Check sheet for the modelled part. Datum: model origin and axes. Units: mm. Round coordinates to 2 decimals unless told otherwise and drop trailing zeros. Answer in a Markdown table with one row per item.
```python
from build123d import *
from OCP.BRepFilletAPI import BRepFilletAPI_MakeChamfer

# Parameters (mm, degrees)
SKETCH1_W                       = 140
SKETCH1_H                       = 80
BOSS_EXTRUDE1_DEPTH             = 7
SKETCH3_W                       = 140
SKETCH3_H                       = 80
SKETCH2_W                       = 120
SKETCH2_H                       = 60
CHAMFER1_SIZE                   = 2
SKETCH4_R                       = 2.05
CUT_EXTRUDE1_DEPTH              = 7
SKETCH5_W                       = 114
SKETCH5_H                       = 50
CUT_EXTRUDE2_DEPTH              = 29
SKETCH6_W                       = 114
SKETCH6_H                       = 62
CUT_EXTRUDE3_DEPTH              = 25
SKETCH7_W                       = 6
SKETCH7_H                       = 62
CUT_EXTRUDE4_DEPTH              = 4
SKETCH8_R                       = 2.05
CUT_EXTRUDE5_DEPTH              = 6
CHAMFER2_SIZE                   = 1
CHAMFER2_SIZE2                  = 0.471497246
CHAMFER3_SIZE                   = 0.6
SKIZZE1_W                       = 54.050484576
SKIZZE1_H                       = 7.5
SKIZZE1_W_2                     = 4
SKIZZE1_H_2                     = 21.453027382
AUFSATZ_LINEAR_AUSTRAGEN1_DEPTH = 10
SKIZZE3_W                       = 29.974757712
SKIZZE3_H                       = 3
SCHNITT_LINEAR_AUSTRAGEN2_DEPTH = 4


with BuildPart() as part:
    # Sketch1 → Boss-Extrude1 (new body)
    with BuildSketch(Plane(origin=(0, 0, 0), x_dir=(1, 0, 0), z_dir=(0, 1, 0))):
        Rectangle(SKETCH1_W, SKETCH1_H)
    extrude(amount=BOSS_EXTRUDE1_DEPTH)

    # Sketch3 → Loft2 section 0
    with BuildSketch(Plane(origin=(0, 7, 0), x_dir=(1, 0, 0), z_dir=(0, 1, 0))):
        Rectangle(SKETCH3_W, SKETCH3_H)
    # Sketch2 → Loft2 section 1
    with BuildSketch(Plane(origin=(0, 30, 0), x_dir=(1, 0, 0), z_dir=(0, 1, 0))):
        Rectangle(SKETCH2_W, SKETCH2_H)
    loft()

    # Chamfer1
    chamfer1_edges = [part.edges().sort_by_distance(p)[0] for p in [
        (-70, 3.5, 40),
        (70, 3.5, 40),
        (70, 3.5, -40),
        (-70, 3.5, -40),
    ]]
    chamfer(chamfer1_edges, length=CHAMFER1_SIZE)

    # Sketch4 → Cut-Extrude1 (cut)
    with BuildSketch(Plane.XZ):
        with Locations(Location((40, -36.5, 0), (0, 0, 270))):
            Circle(SKETCH4_R)
        with Locations(Location((-40, -36.5, 0), (0, 0, 270))):
            Circle(SKETCH4_R)
    cut_extrude1 = extrude(amount=-CUT_EXTRUDE1_DEPTH, mode=Mode.SUBTRACT)

    # Sketch5 → Cut-Extrude2 (cut)
    with BuildSketch(Plane.XZ):
        Rectangle(SKETCH5_W, SKETCH5_H)
    extrude(amount=-CUT_EXTRUDE2_DEPTH, mode=Mode.SUBTRACT)

    # Mirror1: Cut-Extrude1 across plane
    add(cut_extrude1.mirror(Plane.XY), mode=Mode.SUBTRACT)

    # Sketch6 → Cut-Extrude3 (cut)
    with BuildSketch(Plane.XZ):
        Rectangle(SKETCH6_W, SKETCH6_H)
    extrude(amount=-CUT_EXTRUDE3_DEPTH, mode=Mode.SUBTRACT)

    # Sketch7 → Cut-Extrude4 (cut)
    with BuildSketch(Plane.XZ):
        with Locations((-60, 0)):
            Rectangle(SKETCH7_W, SKETCH7_H)
        with Locations((60, 0)):
            Rectangle(SKETCH7_W, SKETCH7_H)
    extrude(amount=-CUT_EXTRUDE4_DEPTH, mode=Mode.SUBTRACT)

    # Sketch8 → Cut-Extrude5 (cut)
    with BuildSketch(Plane.XZ.offset(-4)):
        with Locations(Location((-60, 25, 0), (0, 0, 270))):
            Circle(SKETCH8_R)
        with Locations(Location((-60, -25, 0), (0, 0, 270))):
            Circle(SKETCH8_R)
        with Locations(Location((60, -25, 0), (0, 0, 90))):
            Circle(SKETCH8_R)
        with Locations(Location((60, 25, 0), (0, 0, 90))):
            Circle(SKETCH8_R)
    extrude(amount=-CUT_EXTRUDE5_DEPTH, mode=Mode.SUBTRACT)

    # Chamfer2: one chamfer whose edges measure the first distance from different faces: ONE call of the kernel's chamfer builder (chamfer() names one face for all edges)
    chamfer2_edges_1 = [part.edges().sort_by_distance(p)[0] for p in [
        (60, 30, 0),
    ]]
    chamfer2_side_1 = [part.faces().sort_by_distance(p)[0] for p in [
        (65.225405922, 17.98156638, 0),
    ]]
    chamfer2_edges_2 = [part.edges().sort_by_distance(p)[0] for p in [
        (0, 30, -30),
    ]]
    chamfer2_side_2 = [part.faces().sort_by_distance(p)[0] for p in [
        (0, 18.221212121, -35.121212121),
    ]]
    chamfer2_edges_3 = [part.edges().sort_by_distance(p)[0] for p in [
        (-60, 30, 0),
    ]]
    chamfer2_side_3 = [part.faces().sort_by_distance(p)[0] for p in [
        (-65.225405922, 17.98156638, 0),
    ]]
    chamfer2_edges_4 = [part.edges().sort_by_distance(p)[0] for p in [
        (0, 30, 30),
    ]]
    chamfer2_side_4 = [part.faces().sort_by_distance(p)[0] for p in [
        (0, 18.221212121, 35.121212121),
    ]]
    chamfer2 = BRepFilletAPI_MakeChamfer(part.part.solid().wrapped)
    for e in chamfer2_edges_1:
        chamfer2.Add(CHAMFER2_SIZE, CHAMFER2_SIZE2, e.wrapped, chamfer2_side_1[0].wrapped)  # the first distance lies on this face
    for e in chamfer2_edges_2:
        chamfer2.Add(CHAMFER2_SIZE, CHAMFER2_SIZE2, e.wrapped, chamfer2_side_2[0].wrapped)  # the first distance lies on this face
    for e in chamfer2_edges_3:
        chamfer2.Add(CHAMFER2_SIZE, CHAMFER2_SIZE2, e.wrapped, chamfer2_side_3[0].wrapped)  # the first distance lies on this face
    for e in chamfer2_edges_4:
        chamfer2.Add(CHAMFER2_SIZE, CHAMFER2_SIZE2, e.wrapped, chamfer2_side_4[0].wrapped)  # the first distance lies on this face
    add(Compound.cast(chamfer2.Shape()), mode=Mode.REPLACE)

    # Chamfer3
    chamfer3_edges = [part.edges().sort_by_distance(p)[0] for p in [
        (0, 0, 40),
        (70, 0, 0),
        (-70, 0, 0),
        (0, 0, -40),
        (-69, 0, -39),
        (69, 0, -39),
        (69, 0, 39),
        (-69, 0, 39),
    ]]
    chamfer(chamfer3_edges, length=CHAMFER3_SIZE)

    # Skizze1 → Aufsatz-Linear austragen1 (add)
    with BuildSketch(Plane.XZ.offset(-29)):
        with Locations((0, -21.25)):
            Rectangle(SKIZZE1_W, SKIZZE1_H)
        with Locations((0, 21.25)):
            Rectangle(SKIZZE1_W, SKIZZE1_H)
        with Locations((55, 0)):
            Rectangle(SKIZZE1_W_2, SKIZZE1_H_2)
    extrude(amount=AUFSATZ_LINEAR_AUSTRAGEN1_DEPTH)

    # Skizze3 → Schnitt-Linear austragen2 (cut)
    with BuildSketch(Plane(origin=(0, 29, 0), x_dir=(-1, 0, 0), z_dir=(0, -1, 0))):
        with Locations((42.012621144, -26.5)):
            Rectangle(SKIZZE3_W, SKIZZE3_H)
        with Locations((-42.012621144, -26.5)):
            Rectangle(SKIZZE3_W, SKIZZE3_H)
        with Locations((42.012621144, 26.5)):
            Rectangle(SKIZZE3_W, SKIZZE3_H)
        with Locations((-42.012621144, 26.5)):
            Rectangle(SKIZZE3_W, SKIZZE3_H)
    extrude(amount=SCHNITT_LINEAR_AUSTRAGEN2_DEPTH, mode=Mode.SUBTRACT)


solid = part.part
```
(1) Scan lines: probe 1 along X at (y, z) = (5.95, 25); probe 2 along X at (y, z) = (4, -36.5); probe 3 along Z at (x, y) = (60, 6.7). Record each from-to range of solid material in increasing order. Write a range as from..to.
Solutions:
| item | result |
|---|---|
| probe 1 | -70..-62.05, -57.95..-57, 57..57.95, 62.05..70 |
| probe 2 | -70..-42.05, -37.95..37.95, 42.05..70 |
| probe 3 | -40..-27.05, -22.95..22.95, 27.05..40 |
(2) Section check A-A on y = 23. Give the number of separate pieces and of enclosed holes in the cut face, plus the area to 3 significant figures.
Solutions:
| item | result |
|---|---|
| separate pieces | 3 |
| enclosed holes | 1 |
| area | 2,160 mm^2 |
(3) Depth check by flat-ended pin: pin 1 Ø2 at (x, y) = (-25.5, 21) entering from -Z; pin 2 Ø4.5 at (x, z) = (60.5, -25.5) entering from -Y; pin 3 Ø6 at (x, z) = (-15.5, 2.5) entering from -Y. Enter the tip coordinate at first touch or a pass-through.
Solutions:
| item | result |
|---|---|
| pin 1 | z = -34.35 |
| pin 2 | y = 4 |
| pin 3 | y = 29 |
(4) Draft check along X on faces 1 (the flat face through (-1, 30, 0)), 2 (the flat face through (-27.025, 24, -22)), 3 (the flat face through (-70, 4, 1)), 4 (the flat face through (70, 4, 1)). Enter one of: pulls with the +X half, pulls with the -X half, needs draft (parallel to the pull), parting line crosses it, or undercut.
Solutions:
| item | result |
|---|---|
| face 1 | needs draft |
| face 2 | undercut |
| face 3 | pulls with the -X half |
| face 4 | pulls with the +X half |
